Check sheet for the drawn part. Datum: minimum x, y, z corner. Units: mm. Round coordinates to 2 decimals unless told otherwise and drop trailing zeros. Write each loop counter-clockwise with the first axis right and the second up, starting at its lowest first coordinate (ties: lowest second). Pieces come first, ordered by that corner, then holes. Notation, with made-up numbers: (56, -15.5) -> (70, -15.5) arc R23 ccw to (70, -0.5) -> close; hole circle Ø7 at (-15, -8). An arc over 180 degrees is marked (long way). Use CSV: the item, a comma, the result in double quotes.
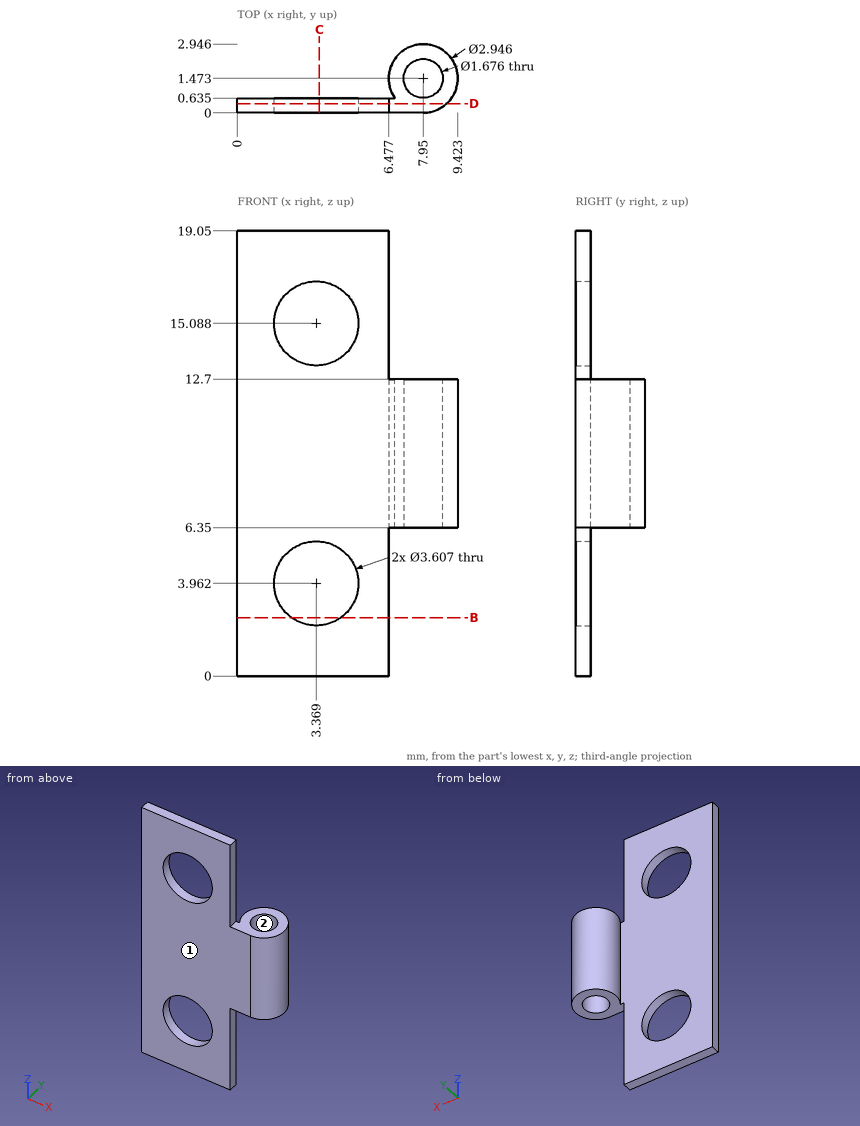
Q1. Material ranges on L1, parallel to Z at x = 3.5, y = 0.45; L2, parallel to Y at x = 2, z = 9.5 (1 decimal); L3, parallel to Z at x = 8.5, y = 0.5, recorded low to high.
Filled in:
L1,"0 to 2.16, 5.76 to 13.29, 16.89 to 19.05"
L2,"0 to 0.6"
L3,"6.35 to 12.7"
Q2. Go/stop test with flat-tipped pins: P1, Ø2, axis at x = 7.5, z = 9, coming from the +Y side; P2, Ø4, axis at x = 3.5, z = 11.5, coming from the +Y side (3 decimals); P3, Ø0.7, axis at y = 0, z = 14.5, coming from the +X side; P4, Ø1.5, axis at x = 8.5, y = 1, coming from the +Z side. Record where each tip stops, or that it passes through.
Filled in:
P1,"y = 2.95"
P2,"y = 0.635"
P3,"x = 6.48"
P4,"z = 12.7"
Q3. Mould release check, pull along X, two halves, no side actions. Record for the marked faces 1 and 2: released by +X, released by -X, zero draft, split by the parting line, or undercut.
Filled in:
face 1,"zero draft"
face 2,"undercut"
Q4. Section check B-B (z = 2.5). Record the cut outline in (x, y) (1 decimal).
Filled in:
outline,"(0, 0) -> (2.3, 0) -> (2.3, 0.6) -> (0, 0.6) -> close; (4.4, 0) -> (6.5, 0) -> (6.5, 0.6) -> (4.4, 0.6) -> close"
Q5. Section check D-D (y = 0.4). Record the cut outline in (x, z).
Filled in:
outline,"(0, 0) -> (6.48, 0) -> (6.48, 6.35) -> (8.96, 6.35) -> (8.96, 12.7) -> (6.48, 12.7) -> (6.48, 19.05) -> (0, 19.05) -> close; hole circle Ø3.61 at (3.37, 3.96); hole circle Ø3.61 at (3.37, 15.09)"
Q6. Section check C-C (x = 3.5). State how many separate pieces and enclosed holes the cut face has.
Filled in:
separate pieces,"3"
enclosed holes,"0"
